```python
from build123d import *

# Parameters (mm, degrees)
SKETCH_1_W                         = 100
SKETCH_1_H                         = 25
SM_BASE_FLANGE_1_DEPTH             = 2
SM_EDGE_FLANGE_1_STRIP_W           = 11
SM_EDGE_FLANGE_1_STRIP_H           = 2
SM_EDGE_FLANGE_1_STRIP_CUT_DEPTH   = 100
SM_EDGE_FLANGE_1_STRIP_2_W         = 11
SM_EDGE_FLANGE_1_STRIP_2_H         = 2
SM_EDGE_FLANGE_1_STRIP_CUT_2_DEPTH = 100
SM_EDGE_FLANGE_1_DEPTH             = 100
SM_EDGE_FLANGE_1_BEND_DEPTH        = 100
SKETCH_12_W                        = 25
SKETCH_12_H                        = 25
CUT_EXTRUDE_1_DEPTH                = 4
SKETCH_24_W                        = 24
SKETCH_24_H                        = 4
EXTRUDE_1_DEPTH                    = 2


# Sheet-metal steps are written as plain solids
with BuildPart() as part:
    # Sketch 1 → Базовая кромка1 (new body)
    with BuildSketch(Plane.XY):
        Rectangle(SKETCH_1_W, SKETCH_1_H)
    extrude(amount=-SM_BASE_FLANGE_1_DEPTH)

    # Ребро-кромка1 strip (across the edge) → Ребро-кромка1 strip cut (cut)
    with BuildSketch(Plane(origin=(-50, 12.5, -2), x_dir=(0, -1, 0), z_dir=(1, 0, 0))):
        with Locations((-4, -1)):
            Rectangle(SM_EDGE_FLANGE_1_STRIP_W, SM_EDGE_FLANGE_1_STRIP_H)
    extrude(amount=SM_EDGE_FLANGE_1_STRIP_CUT_DEPTH, mode=Mode.SUBTRACT)

    # Ребро-кромка1 strip 2 (across the edge) → Ребро-кромка1 strip cut 2 (cut)
    with BuildSketch(Plane(origin=(50, -12.5, -2), x_dir=(0, 1, 0), z_dir=(-1, 0, 0))):
        with Locations((-4, -1)):
            Rectangle(SM_EDGE_FLANGE_1_STRIP_2_W, SM_EDGE_FLANGE_1_STRIP_2_H)
    extrude(amount=SM_EDGE_FLANGE_1_STRIP_CUT_2_DEPTH, mode=Mode.SUBTRACT)

    # Ребро-кромка1 section (across the edge) → Ребро-кромка1 (add)
    with BuildSketch(Plane(origin=(-50, 12.5, -2), x_dir=(0, -1, 0), z_dir=(1, 0, 0))):
        with BuildLine():
            Line((-2, 1.5), (-2, 23))
            Line((-2, 23), (0, 23))
            Line((0, 23), (0, 1.5))
            ThreePointArc((0, 1.5), (0.439339828, 0.439339828), (1.5, 0))
            Line((1.5, 0), (1.5, -2))
            ThreePointArc((1.5, -2), (-0.974873734, -0.974873734), (-2, 1.5))
        make_face()
    extrude(amount=SM_EDGE_FLANGE_1_DEPTH)

    # Ребро-кромка1 section 2 (across the edge) → Ребро-кромка1 bend (add)
    with BuildSketch(Plane(origin=(50, -12.5, -2), x_dir=(0, 1, 0), z_dir=(-1, 0, 0))):
        with BuildLine():
            Line((-2, 1.5), (-2, 23))
            Line((-2, 23), (0, 23))
            Line((0, 23), (0, 1.5))
            ThreePointArc((0, 1.5), (0.439339828, 0.439339828), (1.5, 0))
            Line((1.5, 0), (1.5, -2))
            ThreePointArc((1.5, -2), (-0.974873734, -0.974873734), (-2, 1.5))
        make_face()
    extrude(amount=SM_EDGE_FLANGE_1_BEND_DEPTH)

    # Эскиз12 → Вырез-Вытянуть1 (cut)
    with BuildSketch(Plane(origin=(0, 14.5, 0), x_dir=(1, 0, 0), z_dir=(0, 1, 0))):
        with Locations((0, 12.5)):
            Rectangle(SKETCH_12_W, SKETCH_12_H)
    extrude(amount=-CUT_EXTRUDE_1_DEPTH, mode=Mode.SUBTRACT)

    # Эскиз24 → Бобышка-Вытянуть1 (add)
    with BuildSketch(Plane.XY):
        with Locations((0, 12.5)):
            Rectangle(SKETCH_24_W, SKETCH_24_H)
    extrude(amount=-EXTRUDE_1_DEPTH)


solid = part.part
```
Design review of the part built by this model. Coordinates are the model's own, in mm. A direction names the side the tool comes from. Coordinates: 2 decimals unless noted, no trailing zeros. Write each loop counter-clockwise with the first axis right and the second up, starting at its lowest first coordinate (ties: lowest second). Pieces come first, ordered by that corner, then holes. Notation, with made-up numbers: M 89,-26.75 L 128,-26.75 A14 ccw 128,-17.75 Z; hole C 52,72.5 d2. An arc over 180 degrees is marked long. Answer as a JSON object with one key per item and string values.
Item 1: Draft analysis for pull direction Y (two halves, no side actions). For faces 6 (the cylindrical face through (30.99, 13.45, -1)), 7 (the cylindrical face through (0.7, -13.45, -1)), 8 (the flat face through (-32, 12.5, -14)), 9 (the flat face through (-1, 2, 0)), state which applies: pulls with the +Y half, pulls with the -Y half, needs draft (parallel to the pull), parting line crosses it, or undercut.
Outcome:
{"face 6": "pulls with the +Y half", "face 7": "pulls with the -Y half", "face 8": "undercut", "face 9": "needs draft"}
Item 2: Add section B-B, the plane x = 37. Give the boundary of the cut face in (y, z), and give its area (3 significant figures).
Outcome:
{"outline": "M -14.5,-25 L -12.5,-25 L -12.5,-3.5 A1.5 cw -11,-2 L 11,-2 A1.5 cw 12.5,-3.5 L 12.5,-25 L 14.5,-25 L 14.5,-3.5 A3.5 ccw 11,0 L -11,0 A3.5 ccw -14.5,-3.5 Z", "area": "146 mm²"}
Item 3: Insertion check: pin 1 Ø5 at (x, y) = (14, 0) entering from -Z. The pin has a flat end and moves straight along its axis. Give the tip position at first contact, or say it passes through.
Outcome:
{"pin 1": "z = -2"}
Item 4: Wall thickness on probe 1 along Y at (x, z) = (15.5, -4.75); probe 2 along X at (y, z) = (13, -16); probe 3 along Z at (x, y) = (31, -9): over which ranges is each line inside the solid? List them lowest first.
Outcome:
{"probe 1": "-14.5 to -12.5, 12.5 to 14.5", "probe 2": "-50 to -12.5, 12.5 to 50", "probe 3": "-2 to 0"}
Item 5: Add section A-A, the plane z = -22.5. Give the boundary of the cut face in (x, y).
Outcome:
{"outline": "M -50,-14.5 L 50,-14.5 L 50,-12.5 L -50,-12.5 Z; M -50,12.5 L -12.5,12.5 L -12.5,14.5 L -50,14.5 Z; M 12.5,12.5 L 50,12.5 L 50,14.5 L 12.5,14.5 Z"}
Item 6: Add section C-C, the plane y = 2. Give the boundary of the cut face in (x, z).
Outcome:
{"outline": "M -50,-2 L 50,-2 L 50,0 L -50,0 Z"}
Item 7: Machinability: for faces 1 (the flat face through (31, 12.5, -14)), 2 (the flat face through (50, 0, -1)), 3 (the flat face through (12.5, 13, -12)), 4 (the cylindrical face through (-31.51, 13.45, -1)), 5 (the flat face through (31, 14.5, -14)), which of the approach directions +Z, -Z, +X, -X, +Y, -Y give a long, thin tool a straight path to every point of the face, cutting with its end or side? Answer none if there is none.
Outcome:
{"face 1": "-Z, +X, -X", "face 2": "+Z, -Z, +X, +Y, -Y", "face 3": "+Z, -Z, +Y", "face 4": "+Z, -X, +Y", "face 5": "+Z, -Z, +X, -X, +Y"}
